Model file for the job. Use its own axes, mm. Face numbers are marked on the shaded views. Round coordinates to 2 decimals unless told otherwise and drop trailing zeros. Loops run counter-clockwise (first coordinate to the right, second up) from the corner with the lowest first, then second, coordinate; pieces in that order, holes last. Notation, with made-up numbers: M -32,-18 L -23,-18 A12 ccw -23,0 Z; hole C 88.25,49.25 d3. An arc over 180 degrees is marked long. Answer in a Markdown table with one row per item.
from build123d import *

# Parameters (mm, degrees)
EXTRUDE_1_DEPTH     = 4
CUT_EXTRUDE_1_DEPTH = 3
SKETCH_5_R          = 1.25
CUT_EXTRUDE_2_DEPTH = 12.4
SKETCH_6_W          = 17
SKETCH_6_H          = 35
EXTRUDE_2_DEPTH     = 4
SKETCH_7_W          = 13
SKETCH_7_H          = 24
CUT_EXTRUDE_3_DEPTH = 12.1
SKETCH_8_W          = 4
SKETCH_8_H          = 4
SKETCH_8_R          = 1.175
EXTRUDE_3_DEPTH     = 15
EXTRUDE_4_DEPTH     = 5
SKETCH_10_R         = 1.175
CUT_EXTRUDE_4_DEPTH = 12.7


with BuildPart() as part:
    # 草圖1 → 填料-伸長1 (new body)
    with BuildSketch(Plane.XY):
        with BuildLine():
            Line((7.5, 0), (7.5, 52))
            ThreePointArc((7.5, 52), (0, 59.5), (-7.5, 52))
            Line((-7.5, 52), (-7.5, 0))
            Line((-7.5, 0), (7.5, 0))
        make_face()
    extrude(amount=EXTRUDE_1_DEPTH)

    # 草圖3 → 除料-伸長1 (cut)
    with BuildSketch(Plane.XY):
        with BuildLine():
            ThreePointArc((-2.132795501, 52), (0, 54.132795501), (2.132795501, 52))
            Line((2.132795501, 52), (5, 34.5))
            Line((5, 34.5), (2.114741289, 16.658021353))
            ThreePointArc((2.114741289, 16.658021353), (-0.171540182, 14.864665347), (-2.142213835, 17))
            Line((-2.142213835, 17), (-5, 34.5))
            Line((-5, 34.5), (-2.132795501, 52))
        make_face()
    extrude(amount=CUT_EXTRUDE_1_DEPTH, mode=Mode.SUBTRACT)

    # 草圖5 → 除料-伸長2 (cut)
    with BuildSketch(Plane.XY):
        with Locations((0, 34.5)):
            Circle(SKETCH_5_R)
    extrude(amount=CUT_EXTRUDE_2_DEPTH, mode=Mode.SUBTRACT)

    # 草圖6 → 填料-伸長2 (add)
    with BuildSketch(Plane.XY):
        with Locations((0, -17.5)):
            Rectangle(SKETCH_6_W, SKETCH_6_H)
    extrude(amount=EXTRUDE_2_DEPTH)

    # 草圖7 → 除料-伸長3 (cut)
    with BuildSketch(Plane.XY):
        with Locations((0, -18)):
            Rectangle(SKETCH_7_W, SKETCH_7_H)
    extrude(amount=CUT_EXTRUDE_3_DEPTH, mode=Mode.SUBTRACT)

    # 草圖8 → 填料-伸長3 (add)
    with BuildSketch(Plane.XY):
        with Locations((0, -4)):
            Rectangle(SKETCH_8_W, SKETCH_8_H)
        with Locations((0, -4)):
            Circle(SKETCH_8_R, mode=Mode.SUBTRACT)
    extrude(amount=-EXTRUDE_3_DEPTH)

    # 草圖9 → 填料-伸長4 (add)
    with BuildSketch(Plane(origin=(0, -35, 0), x_dir=(1, 0, 0), z_dir=(0, 1, 0))):
        Polygon((-8.5, 0), (-5, 0), (-5, 5), (5, 5), (5, 0), (8.5, 0), (8.5, 15), (-8.5, 15), align=None)
    extrude(amount=EXTRUDE_4_DEPTH)

    # 草圖10 → 除料-伸長4 (cut)
    with BuildSketch(Plane(origin=(0, 0, -15), x_dir=(-1, 0, 0), z_dir=(0, 0, -1))):
        with Locations((0, -32.5)):
            Circle(SKETCH_10_R)
    extrude(amount=-CUT_EXTRUDE_4_DEPTH, mode=Mode.SUBTRACT)


solid = part.part
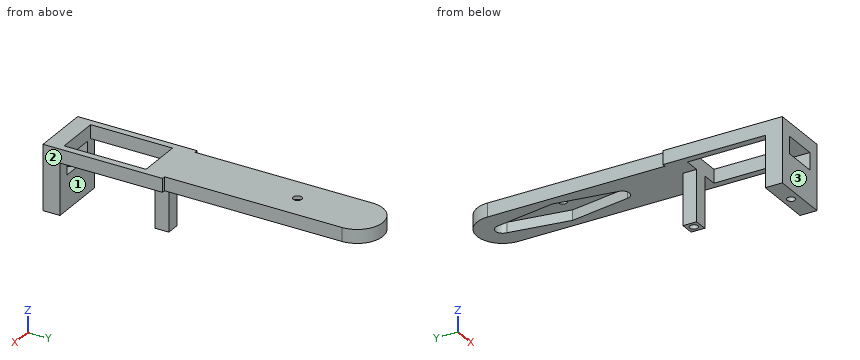
1. Saw through at C-C (y = -19). Write the cut outline in (x, z), and give its area (3 significant figures).
Verdict:
| item | result |
|---|---|
| outline | M -8.5,0 L -6.5,0 L -6.5,4 L -8.5,4 Z; M 6.5,0 L 8.5,0 L 8.5,4 L 6.5,4 Z |
| area | 16.0 mm² |
2. Wall check: probe 1 along Y at (x, z) = (0, 3.5); probe 2 along Y at (x, z) = (0, -10) (3 decimals); probe 3 along Y at (x, z) = (-0.5, -13.25). Give the ranges that are in metal, low to high.
Verdict:
| item | result |
|---|---|
| probe 1 | y = -35 to -30, -6 to 33.25, 35.75 to 59.5 |
| probe 2 | y = -35 to -33.675, -31.325 to -30, -6 to -5.175, -2.825 to -2 |
| probe 3 | y = -35 to -33.56, -31.44 to -30, -6 to -5.06, -2.94 to -2 |
3. Saw through at B-B (x = 0). State how many separate pieces and enclosed holes the cut face has, and give its area (3 significant figures).
Verdict:
| item | result |
|---|---|
| separate pieces | 5 |
| enclosed holes | 0 |
| area | 213 mm² |
4. Mould opens along Y. For the marked faces 1, 2 and 3 say: +Y half, -Y half, draft (parallel to the pull), parting line (faces both ways), or undercut.
Verdict:
| item | result |
|---|---|
| face 1 | undercut |
| face 2 | draft |
| face 3 | -Y half |
5. Pin check, flat tips, straight feed: pin 1 (4 mm diameter, centred on x = -0.5, z = -4.5, fed in from +Y); pin 2 (2 mm diameter, centred on x = -6.5, z = -3.5, fed in from +Y); pin 3 (4.5 mm diameter, centred on y = -4.5, z = -6, fed in from +X); pin 4 (1.5 mm diameter, centred on x = 0, y = 34.5, fed in from +Z). Stop position of each tip, or through.
Verdict:
| item | result |
|---|---|
| pin 1 | stops at y = -2 |
| pin 2 | stops at y = -30 |
| pin 3 | stops at x = 2 |
| pin 4 | passes through |
6. Saw through at D-D (z = -8.5). Write the cut outline in (x, y) (3 decimals).
Verdict:
| item | result |
|---|---|
| outline | M -8.5,-35 L 8.5,-35 L 8.5,-30 L -8.5,-30 Z; M -2,-6 L 2,-6 L 2,-2 L -2,-2 Z; hole C 0,-32.5 d2.35; hole C 0,-4 d2.35 |
7. Saw through at A-A (z = -1.75). Write the cut outline in (x, y) (3 decimals).
Verdict:
| item | result |
|---|---|
| outline | M -8.5,-35 L -5,-35 L -5,-30 L -8.5,-30 Z; M -2,-6 L 2,-6 L 2,-2 L -2,-2 Z; M 5,-35 L 8.5,-35 L 8.5,-30 L 5,-30 Z; hole C 0,-4 d2.35 |
